```python
from build123d import *

# Parameters (mm, degrees)
PAD_DEPTH    = 1.5
SKETCH001_R  = 3.8
PAD001_DEPTH = 5
SKETCH002_R  = 2.6
POCKET_DEPTH = 5.5
FILLET_R     = 0.6
CHAMFER_SIZE = 0.4


with BuildPart() as part:
    # Sketch → Pad (new body)
    with BuildSketch(Plane.XY):
        with BuildLine():
            Line((0.715008, 0), (18, 0))
            ThreePointArc((18, 0), (23.000017, 5), (18, 10))
            Line((18, 10), (0.631198, 10))
            ThreePointArc((0.631198, 10), (0.184874, 9.815126), (0, 9.368802))
            Line((0, 9.368802), (0, 0.715008))
            ThreePointArc((0, 0.715008), (0.209421, 0.209421), (0.715008, 0))
        make_face()
    extrude(amount=PAD_DEPTH)

    # Sketch001 (on Face8 of Pad) → Pad001 (join)
    with BuildSketch(Plane.XY.offset(1.5)):
        with Locations((18, 5)):
            Circle(SKETCH001_R)
    extrude(amount=PAD001_DEPTH)

    # Sketch002 → Pocket (cut)
    with BuildSketch(Plane.XY.offset(6.5)):
        with Locations((18, 5)):
            Circle(SKETCH002_R)
    extrude(amount=-POCKET_DEPTH, mode=Mode.SUBTRACT)

    # Fillet
    fillet_edges = [part.edges().sort_by_distance(p)[0] for p in [
        (21.8, 5, 4),
        (14.2, 5, 1.5),
        (14.2, 5, 6.5),
    ]]
    fillet(fillet_edges, radius=FILLET_R)

    # Chamfer
    chamfer_edges = [part.edges().sort_by_distance(p)[0] for p in [
        (13.6, 5, 1.5),
        (9.357504, 0, 1.5),
        (0.209421, 0.209421, 1.5),
        (23.000017, 5, 1.5),
        (0, 5.041905, 1.5),
        (9.315599, 10, 1.5),
        (0.184874, 9.815126, 1.5),
    ]]
    chamfer(chamfer_edges, length=CHAMFER_SIZE)


solid = part.part
```
For this review, take the finished solid that the model builds, in its own axes (mm). A direction names the side the tool comes from. Coordinates: 2 decimals unless noted, no trailing zeros. Write each loop counter-clockwise with the first axis right and the second up, starting at its lowest first coordinate (ties: lowest second). Pieces come first, ordered by that corner, then holes.
(1) Add section D-D on z = 0.5. Give the boundary of the cut face in (x, y) (3 decimals), then the cut area to 3 significant figures.
(2) For pin 1 Ø2 at (y, z) = (1, 4.5) entering from +X; pin 2 Ø2.5 at (x, y) = (17.5, 4.5) entering from +Z, all flat-tipped, find the tip position at first contact; note any pin that passes through.
(3) Add section A-A on y = 5. Give the boundary of the cut face in (x, z), then the cut area to 3 significant figures.
(4) The part is to be moulded in two halves that separate along Y. For faces 1 (the face through (20.48, 5.78, 3.79)), 2 (the face through (18, 8, 6.5)), 3 (the face through (9.2, 0, 0.5)), 4 (the face through (23, 4.9, 0.5)), say which applies: +Y half, -Y half, draft (parallel to the pull), parting line (faces both ways), or undercut.
(5) Add section C-C on x = 3.5. Give the boundary of the cut face in (y, z), then the cut area to 3 significant figures.
(6) Add section B-B on z = 2.75. Give the boundary of the cut face in (x, y), then the cut area to 3 significant figures.
(7) Tool access review of faces 5 (the face through (9.4, 10, 0.5)), 6 (the face through (14.204, 5.167, 3.973)): name each direction out of +Z, -Z, +X, -X, +Y, -Y from which nothing blocks a thin tool from reaching the whole face with its end or side.
(8) Wall thickness on probe 1 along Y at (x, z) = (18, 4); probe 2 along Z at (x, y) = (4.5, 5.5); probe 3 along X at (y, z) = (6.5, 3.5): over which ranges is each line inside the solid? List them lowest first.
Answer sheet:
1. outline: (0, 0.715) arc R0.715 ccw to (0.715, 0) - (18, 0) arc R5 ccw to (18, 10) - (0.631, 10) arc R0.631 ccw to (0, 9.369) - close
1. area: 219 mm2
2. pin 1: stops at x = 20.33
2. pin 2: stops at z = 1
3. outline: (0, 0) - (23, 0) - (23, 1.1) - (22.6, 1.5) - (22.4, 1.5) arc R0.6 cw to (21.8, 2.1) - (21.8, 5.9) arc R0.6 ccw to (21.2, 6.5) - (20.6, 6.5) - (20.6, 1) - (15.4, 1) - (15.4, 6.5) - (14.8, 6.5) arc R0.6 ccw to (14.2, 5.9) - (14.2, 2.1) arc R0.6 cw to (13.6, 1.5) - (0.4, 1.5) - (0, 1.1) - close
3. area: 43.7 mm2
4. face 1: undercut
4. face 2: draft
4. face 3: -Y half
4. face 4: parting line
5. outline: (0, 0) - (10, 0) - (10, 1.1) - (9.6, 1.5) - (0.4, 1.5) - (0, 1.1) - close
5. area: 14.8 mm2
6. outline: circle Ø7.6 at (18, 5); hole circle Ø5.2 at (18, 5)
6. area: 24.1 mm2
7. face 5: +Z, -Z, +X, -X, +Y
7. face 6: +Z
8. probe 1: y = 1.2 to 2.4, 7.6 to 8.8
8. probe 2: z = 0 to 1.5
8. probe 3: x = 14.51 to 15.88, 20.12 to 21.49
